Work out the finished part from the listing and answer in its coordinate system (mm). A direction names the side the tool comes from. Coordinates: 2 decimals unless noted, no trailing zeros. Order: outer loops, then holes, each group sorted by start corner. A loop starts at its lowest first (then second) coordinate and runs counter-clockwise, first axis right, second up.
1. Find the intervals of material crossed by probe 1 along X at (y, z) = (0.1, 5.25); probe 2 along X at (y, z) = (0.45, 4.5); probe 3 along Y at (x, z) = (-7, -4.75), in increasing order.
2. The part is cut by section B-B, the plane z = 2.5. Give the vertices of the cut face in (x, y), then the cut area to 3 significant figures.
3. Determine the mould class of faces 1 (the flat face through (-2.03, 1.35, 1.79)), 2 (the flat face through (0, 0, 0)), 3 (the cylindrical face through (-19.84, 0.49, 4.88)) for opening direction Z: +Z half, -Z half, draft (parallel to the pull), parting line (faces both ways), or undercut.
4. A flat-ended cylindrical pin translates along its axis: pin 1 Ø3 at (x, z) = (-16, -4.5) entering from -Y. Find the tip coordinate at first contact, or state that the pin passes through.
5. The part is cut by section A-A, the plane z = -5. Give the vertices of the cut face in (x, y), then the cut area to 3 significant figures.
6. The part is cut by section C-C, the plane x = 3. Give the vertices of the cut face in (y, z), then the cut area to 3 significant figures.
7. A tool of negligible diameter and unlimited length cuts with its end or side. For faces 4 (the flat face through (-2.08, 1.35, -2.06)), 5 (the flat face through (1.82, 1.35, 1.74)), 6 (the flat face through (1.77, 1.35, -2.11)), 7 (the flat face through (21.5, 0.5, 0.1)), 8 (the flat face through (-0.3, 0.5, 6)), from which of +Z, -Z, +X, -X, +Y, -Y can it reach the whole face along a straight path? Write none if from no direction.
```python
from build123d import *

# Parameters (mm, degrees)
SKETCH1_W           = 43
SKETCH1_H           = 12
SKETCH1_R           = 0.7
BOSS_EXTRUDE1_DEPTH = 1
BOSS_EXTRUDE2_DEPTH = 0.7


with BuildPart() as part:
    # Sketch1 → Boss-Extrude1 (new body)
    with BuildSketch(Plane(origin=(0, 0, 0), x_dir=(1, 0, 0), z_dir=(0, 1, 0))):
        Rectangle(SKETCH1_W, SKETCH1_H)
        with Locations(Location((-20.534424833, -4.967025936, 0), (0, 0, 270))):
            Circle(SKETCH1_R, mode=Mode.SUBTRACT)
        with Locations(Location((20.465575167, -4.967025936, 0), (0, 0, 270))):
            Circle(SKETCH1_R, mode=Mode.SUBTRACT)
        with Locations(Location((20.465575167, 5.032974064, 0), (0, 0, 270))):
            Circle(SKETCH1_R, mode=Mode.SUBTRACT)
        with Locations(Location((-20.534424833, 5.032974064, 0), (0, 0, 270))):
            Circle(SKETCH1_R, mode=Mode.SUBTRACT)
    extrude(amount=BOSS_EXTRUDE1_DEPTH)

    # Sketch3 → Boss-Extrude2 (add)
    with BuildSketch(Plane(origin=(0, 1, 0), x_dir=(1, 0, 0), z_dir=(0, 1, 0))):
        Polygon((-3.980927617, 0.159893843), (-0.131379893, 4.009441567), (3.71816783, 0.159893843), (-0.131379893, -3.68965388), align=None)
    extrude(amount=BOSS_EXTRUDE2_DEPTH)


solid = part.part
```
Geometry says:
1. probe 1: x = -21.5 to -21.17, -19.89 to 19.83, 21.11 to 21.5
1. probe 2: x = -21.5 to -21.06, -20.01 to 19.94, 20.99 to 21.5
1. probe 3: y = 0 to 1
2. outline: (-21.5, 0) - (21.5, 0) - (21.5, 1) - (1.06, 1) - (1.06, 1.7) - (-1.32, 1.7) - (-1.32, 1) - (-21.5, 1) - close
2. area: 44.7 mm2
3. face 1: +Z half
3. face 2: draft
3. face 3: undercut
4. pin 1: stops at y = 0
5. outline: (-21.5, 0) - (-21.23, 0) - (-21.23, 1) - (-21.5, 1) - close; (-19.84, 0) - (19.77, 0) - (19.77, 1) - (-19.84, 1) - close; (21.16, 0) - (21.5, 0) - (21.5, 1) - (21.16, 1) - close
5. area: 40.2 mm2
6. outline: (0, -6) - (1, -6) - (1, -0.88) - (1.7, -0.88) - (1.7, 0.56) - (1, 0.56) - (1, 6) - (0, 6) - close
6. area: 13.0 mm2
7. face 4: -Z, -X, +Y
7. face 5: +Z, +X, +Y
7. face 6: -Z, +X, +Y
7. face 7: +Z, -Z, +X, +Y, -Y
7. face 8: +Z, +X, -X, +Y, -Y
